For this review, take the finished solid that the model builds, in its own axes (mm). Face numbers are marked on the shaded views. A direction names the side the tool comes from. Give positions to 0.01 mm unless a question says otherwise; leave off trailing zeros. Order: outer loops, then holes, each group sorted by start corner. A loop starts at its lowest first (then second) coordinate and runs counter-clockwise, first axis right, second up. Notation, with made-up numbers: (59, -20) - (105, -20) arc R19 ccw to (105, 2) - close; hole circle Ø9 at (79.25, 85). An arc over 180 degrees is marked (long way). Use a Markdown table: item, result. Add a question column.
1) We need section A-A on z = 8.5. Write out the cut boundary in (x, y) (3 decimals).
2) Mouldability with a two-part tool opening along X and no side actions: class the marked faces 3, 4 and 5 as released by +X, released by -X, zero draft, split by the parting line, or undercut.
3) Clearance check with a flat-ended pin moving along its axis: P1, Ø9, axis at x = -5, y = 1.5, coming from the +Z side. State where the tip first meets the part, or that it passes through.
4) Machinability: for the marked faces 1 and 2, which of the approach directions +Z, -Z, +X, -X, +Y, -Y give a long, thin tool a straight path to every point of the face, cutting with its end or side? Answer none if there is none.
5) We need section C-C on x = 0. Write out the cut boundary in (y, z) (3 decimals).
6) We need section B-B on y = 16. Write out the cut boundary in (x, z), then the cut area to 3 significant figures.
7) Wall thickness on L1, parallel to X at y = 7, z = 10.75; L2, parallel to Z at x = 9, y = 13.5: over which ranges is each line inside the solid? List them lowest first.
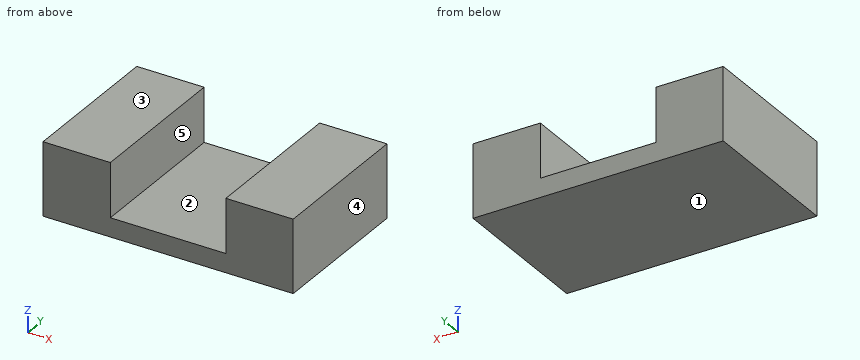
```python
from build123d import *

# Parameters (mm, degrees)
SKETCH1_W           = 65.99377092
SKETCH1_H           = 39.85
BOSS_EXTRUDE1_DEPTH = 20
SKETCH2_W           = 30.48
SKETCH2_H           = 39.85
CUT_EXTRUDE1_DEPTH  = 15.02
SKETCH3_W           = 65.99377092
SKETCH3_H           = 39.85
CUT_EXTRUDE2_DEPTH  = 0.75


with BuildPart() as part:
    # Sketch1 → Boss-Extrude1 (new body)
    with BuildSketch(Plane.XY):
        Rectangle(SKETCH1_W, SKETCH1_H)
    extrude(amount=BOSS_EXTRUDE1_DEPTH)

    # Sketch2 → Cut-Extrude1 (cut)
    with BuildSketch(Plane.XY.offset(20)):
        Rectangle(SKETCH2_W, SKETCH2_H)
    extrude(amount=-CUT_EXTRUDE1_DEPTH, mode=Mode.SUBTRACT)

    # Sketch3 → Cut-Extrude2 (cut)
    with BuildSketch(Plane.XY.offset(20)):
        Rectangle(SKETCH3_W, SKETCH3_H)
    extrude(amount=-CUT_EXTRUDE2_DEPTH, mode=Mode.SUBTRACT)


solid = part.part
```
Checked values:
| question | item | result |
|---|---|---|
| 1 | outline | (-32.997, -19.925) - (-15.24, -19.925) - (-15.24, 19.925) - (-32.997, 19.925) - close; (15.24, -19.925) - (32.997, -19.925) - (32.997, 19.925) - (15.24, 19.925) - close |
| 2 | face 3 | zero draft |
| 2 | face 4 | released by +X |
| 2 | face 5 | undercut |
| 3 | P1 | z = 4.98 |
| 4 | face 1 | -Z, +X, -X, +Y, -Y |
| 4 | face 2 | +Z, +Y, -Y |
| 5 | outline | (-19.925, 0) - (19.925, 0) - (19.925, 4.98) - (-19.925, 4.98) - close |
| 6 | outline | (-33, 0) - (33, 0) - (33, 19.25) - (15.24, 19.25) - (15.24, 4.98) - (-15.24, 4.98) - (-15.24, 19.25) - (-33, 19.25) - close |
| 6 | area | 835 mm² |
| 7 | L1 | -33 to -15.24, 15.24 to 33 |
| 7 | L2 | 0 to 4.98 |
